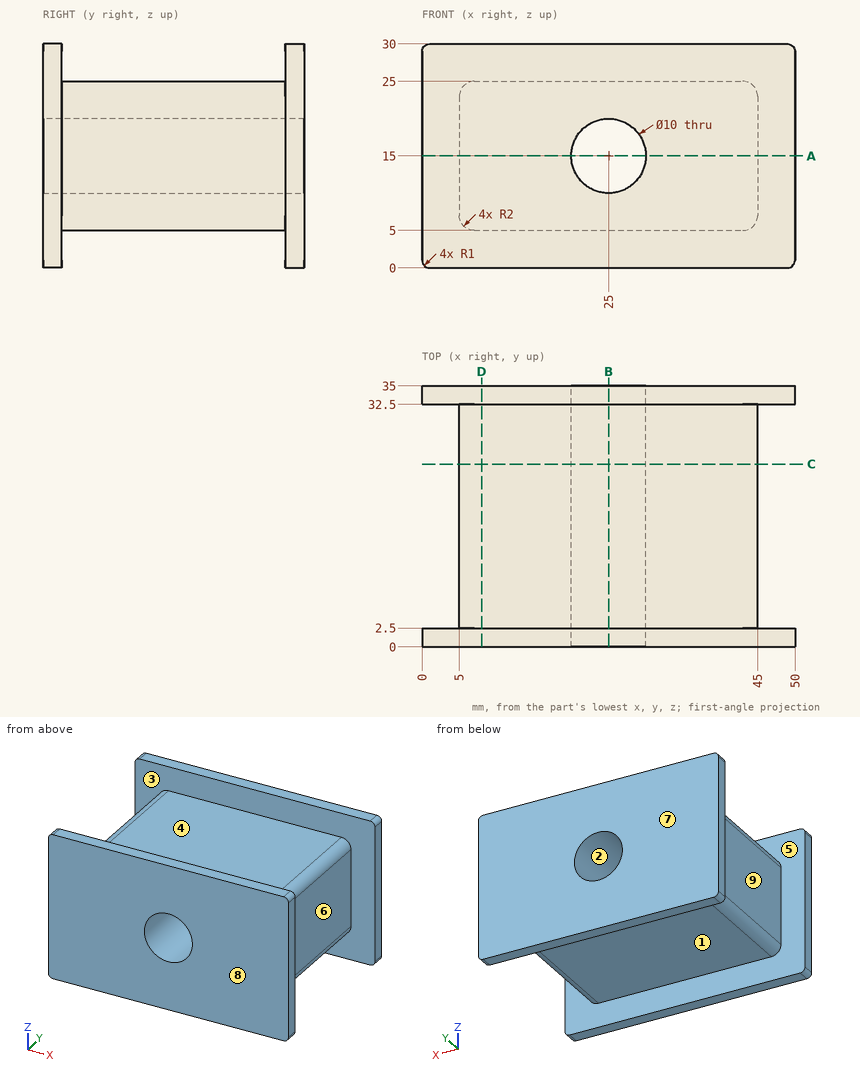
Print and shaded views of the part. All mm, measured from the part's lowest x, y and z. A direction names the side the tool comes from. Give positions to 0.01 mm unless a question says otherwise; leave off trailing zeros. Loops run counter-clockwise (first coordinate to the right, second up) from the corner with the lowest first, then second, coordinate; pieces in that order, holes last. Notation, with made-up numbers: (53, -18.5) - (112, -18.5) arc R29 cw to (112, 16.5) - close; hole circle Ø1 at (88, -27.75). An arc over 180 degrees is marked (long way). Use a Markdown table: item, result.
(1) Pull direction Z, two halves, no side cores. Call the marked faces 1, 2, 3 and 4: +Z half, -Z half, draft (parallel to the pull), parting line (faces both ways), or undercut.
Taken from the geometry:
| item | result |
|---|---|
| face 1 | -Z half |
| face 2 | undercut |
| face 3 | draft |
| face 4 | +Z half |
(2) Band-saw the part on D-D (x = 8). Give the cut face in (y, z).
Taken from the geometry:
| item | result |
|---|---|
| outline | (0, 0) - (2.5, 0) - (2.5, 5) - (32.5, 5) - (32.5, 0) - (35, 0) - (35, 30) - (32.5, 30) - (32.5, 25) - (2.5, 25) - (2.5, 30) - (0, 30) - close |
(3) Band-saw the part on C-C (y = 24.5). Give the cut face in (x, z).
Taken from the geometry:
| item | result |
|---|---|
| outline | (5, 7) arc R2 ccw to (7, 5) - (43, 5) arc R2 ccw to (45, 7) - (45, 23) arc R2 ccw to (43, 25) - (7, 25) arc R2 ccw to (5, 23) - close; hole circle Ø10 at (25, 15) |
(4) Drop flat-ended pins along their axis: pin 1 Ø9 at (x, y) = (30, 16) entering from -Z; pin 2 Ø13 at (y, z) = (10.5, 19) entering from -X; pin 3 Ø13 at (y, z) = (15.5, 17) entering from +X; pin 4 Ø5 at (y, z) = (30.5, 6) entering from -X. Give the stop position or say it passes through.
Taken from the geometry:
| item | result |
|---|---|
| pin 1 | z = 5 |
| pin 2 | x = 5 |
| pin 3 | x = 45 |
| pin 4 | x = 0 |
(5) Band-saw the part on A-A (z = 15). Give the cut face in (x, y).
Taken from the geometry:
| item | result |
|---|---|
| outline | (0, 0) - (20, 0) - (20, 35) - (0, 35) - (0, 32.5) - (5, 32.5) - (5, 2.5) - (0, 2.5) - close; (30, 0) - (50, 0) - (50, 2.5) - (45, 2.5) - (45, 32.5) - (50, 32.5) - (50, 35) - (30, 35) - close |
(6) Wall check: line 1 along Y through (x, z) = (27.5, 4.75); line 2 along X through (y, z) = (23.5, 15); line 3 along Z through (x, y) = (38.5, 7.5). Give the ranges that are in metal, low to high.
Taken from the geometry:
| item | result |
|---|---|
| line 1 | 0 to 2.5, 32.5 to 35 |
| line 2 | 5 to 20, 30 to 45 |
| line 3 | 5 to 25 |
(7) Band-saw the part on B-B (x = 25). Give the cut face in (y, z).
Taken from the geometry:
| item | result |
|---|---|
| outline | (0, 0) - (2.5, 0) - (2.5, 5) - (32.5, 5) - (32.5, 0) - (35, 0) - (35, 10) - (0, 10) - close; (0, 20) - (35, 20) - (35, 30) - (32.5, 30) - (32.5, 25) - (2.5, 25) - (2.5, 30) - (0, 30) - close |
(8) Which spindle directions (+Z, -Z, +X, -X, +Y, -Y) get a long thin tool onto all of the face, cutting with end or side? Do the marked faces 5, 6, 7, 8 and 9. Say none if no direction does.
Taken from the geometry:
| item | result |
|---|---|
| face 5 | none |
| face 6 | +Z, -Z, +X |
| face 7 | +Z, -Z, +X, -X, +Y |
| face 8 | +Z, -Z, +X, -X, -Y |
| face 9 | +Z, -Z, -X |
